from build123d import *

# Parameters (mm, degrees)
SZKIC1_R                    = 1.225
DODANIE_WYCI_GNI_CIE1_DEPTH = 1


with BuildPart() as part:
    # Szkic1 → Dodanie-wyciągnięcie1 (new body)
    with BuildSketch(Plane.XY):
        with BuildLine():
            Line((-7.587614458, 10.373277108), (12.012385542, 10.373277108))
            Line((12.012385542, 10.373277108), (12.012385542, 1.653277108))
            Line((12.012385542, 1.653277108), (14.722385542, 1.653277108))
            ThreePointArc((14.722385542, 1.653277108), (16.341660071, 0.982551637), (17.012385542, -0.636722892))
            Line((17.012385542, -0.636722892), (17.012385542, -0.656722892))
            ThreePointArc((17.012385542, -0.656722892), (16.341660071, -2.27599742), (14.722385542, -2.946722892))
            Line((14.722385542, -2.946722892), (12.012385542, -2.946722892))
            Line((12.012385542, -2.946722892), (12.012385542, -11.646722892))
            Line((12.012385542, -11.646722892), (-7.587614458, -11.646722892))
            Line((-7.587614458, -11.646722892), (-7.587614458, -2.946722892))
            Line((-7.587614458, -2.946722892), (-10.297614458, -2.946722892))
            ThreePointArc((-10.297614458, -2.946722892), (-11.916888987, -2.27599742), (-12.587614458, -0.656722892))
            Line((-12.587614458, -0.656722892), (-12.587614458, -0.636722892))
            ThreePointArc((-12.587614458, -0.636722892), (-11.916888987, 0.982551637), (-10.297614458, 1.653277108))
            Line((-10.297614458, 1.653277108), (-7.587614458, 1.653277108))
            Line((-7.587614458, 1.653277108), (-7.587614458, 10.373277108))
        make_face()
        with Locations((14.722385542, -0.656722892)):
            Circle(SZKIC1_R, mode=Mode.SUBTRACT)
        with Locations(Location((-10.297614458, -0.656722892, 0), (0, 0, 180))):
            Circle(SZKIC1_R, mode=Mode.SUBTRACT)
    extrude(amount=DODANIE_WYCI_GNI_CIE1_DEPTH)


solid = part.part
Could you check a few things on this model? Use its own coordinates, in mm. A direction names the side the tool comes from. Give positions to 0.01 mm unless a question says otherwise; leave off trailing zeros. Write each loop counter-clockwise with the first axis right and the second up, starting at its lowest first coordinate (ties: lowest second). Pieces come first, ordered by that corner, then holes. Notation, with made-up numbers: (61, 31) - (67, 31) arc R24 cw to (67, 42) - close; hole circle Ø10 at (-23, -33). An arc over 180 degrees is marked (long way). Use CSV: the item, a comma, the result in double quotes. Start each with the question number.
Item 1: If I drill on line 1 along X through (y, z) = (-0.75, 0.35); line 2 along X through (y, z) = (-0.25, 0.2); line 3 along X through (y, z) = (-7.25, 0.9), over which ranges is the centre line in solid material (lowest first)?
Item 2: I want a section at A-A, the plane z = 0.2. Please give me the cut outline in (x, y) (3 decimals).
Item 3: I want a section at C-C, the plane y = 4.75. Please give me the cut outline in (x, z).
Item 4: I'm going to push flat-ended pins straight in: pin 1 (1.5 mm diameter, centred on x = 14.72, y = -0.66, fed in from -Z); pin 2 (0.5 mm diameter, centred on x = -8.5, z = 0.5, fed in from -Y); pin 3 (0.5 mm diameter, centred on y = -7.5, z = 0.5, fed in from -X). Where does each tip first touch, or does it pass through?
Item 5: If we mould it in two halves opening along Y, with no side actions, what happens to faces 4 (the face through (-9.074, -0.711, 0.493)), 5 (the face through (16.36, -2.26, 0.49)), 6 (the face through (13.5, -0.6, 0.5)), 7 (the face through (-7.588, 6, 0.5))? For each: pulls with the +Y half, pulls with the -Y half, needs draft (parallel to the pull), parting line crosses it, or undercut.
Item 6: I want a section at B-B, the plane y = 0. Please give me the cut outline in (x, z).
Item 7: For faces 1 (the face through (-9, 1.653, 0.5)), 2 (the face through (-8.9, -2.947, 0.5)), 3 (the face through (12.012, 6.1, 0.5)), which set-ups out of +Z, -Z, +X, -X, +Y, -Y let a thin tool reach every point of the face, with its end or its side?
Findings:
1,line 1,"x = -12.59 to -11.52, -9.08 to 13.5, 15.94 to 17.01"
1,line 2,"x = -12.55 to -11.45, -9.14 to 13.57, 15.88 to 16.98"
1,line 3,"x = -7.59 to 12.01"
2,outline,"(-12.588, -0.657) arc R2.29 ccw to (-10.298, -2.947) - (-7.588, -2.947) - (-7.588, -11.647) - (12.012, -11.647) - (12.012, -2.947) - (14.722, -2.947) arc R2.29 ccw to (17.012, -0.657) - (17.012, -0.637) arc R2.29 ccw to (14.722, 1.653) - (12.012, 1.653) - (12.012, 10.373) - (-7.588, 10.373) - (-7.588, 1.653) - (-10.298, 1.653) arc R2.29 ccw to (-12.588, -0.637) - close; hole circle Ø2.45 at (-10.298, -0.657); hole circle Ø2.45 at (14.722, -0.657)"
3,outline,"(-7.59, 0) - (12.01, 0) - (12.01, 1) - (-7.59, 1) - close"
4,pin 1,"passes through"
4,pin 2,"stops at y = -2.95"
4,pin 3,"stops at x = -7.59"
5,face 4,"undercut"
5,face 5,"pulls with the -Y half"
5,face 6,"undercut"
5,face 7,"needs draft"
6,outline,"(-12.5, 0) - (-11.33, 0) - (-11.33, 1) - (-12.5, 1) - close; (-9.26, 0) - (13.69, 0) - (13.69, 1) - (-9.26, 1) - close; (15.76, 0) - (16.92, 0) - (16.92, 1) - (15.76, 1) - close"
7,face 1,"+Z, -Z, -X, +Y"
7,face 2,"+Z, -Z, -X, -Y"
7,face 3,"+Z, -Z, +X, +Y"
